Can you work these out from the model? Positions are in its coordinate system, mm. A direction names the side the tool comes from. Give positions to 0.01 mm unless a question says otherwise; leave off trailing zeros. Loops run counter-clockwise (first coordinate to the right, second up) from the corner with the lowest first, then second, coordinate; pieces in that order, holes last. Notation, with made-up numbers: (-24, 47.25) - (8, 47.25) arc R24 cw to (8, 76.25) - close; hole circle Ø10 at (-23, -33). An arc over 180 degrees is marked (long way). Write item = value, one per line.
from build123d import *

# Parameters (mm, degrees)
DELETE_START           = -13.5
DELETE_FACE_1_DEPTH    = 27
MOVE_FACE_1_BY         = 7
MOVE_FACE_2_BY         = 5.5
SKETCH_2_W             = 48.263019836
SKETCH_2_H             = 43.058184364
CUT_EXTRUDE_1_DEPTH    = 20
EXTRUDE_1_DEPTH        = 2
EXTRUDE_1_DEPTH_BACK   = 5
SKETCH_3_W             = 20
SKETCH_3_H             = 30
HOLE_WIZARD_M5_1_D     = 4.2
HOLE_WIZARD_M5_1_DEPTH = 20
HOLE_WIZARD_M5_1_TIP   = 1.2618073


with BuildPart() as part:
    # Delete Face 1: read off the stored shape, not the designer's step
    # Delete Face 1 outline → Delete Face 1 (new body)
    with BuildSketch(Plane.YZ.offset(DELETE_START)):
        with BuildLine():
            ThreePointArc((-8.364285714, 23.895568572), (-8.397831007, 23.931741933), (-8.41, 23.979551078))
            Line((-8.41, 23.979551078), (-8.41, 26.020448922))
            ThreePointArc((-8.41, 26.020448922), (-8.397831007, 26.068258067), (-8.364285714, 26.104431428))
            ThreePointArc((-8.364285714, 26.104431428), (-7.725958169, 26.423724028), (-7.033327746, 26.595982314))
            ThreePointArc((-7.033327746, 26.595982314), (-6.723611818, 26.762379014), (-6.6, 27.091517187))
            Line((-6.6, 27.091517187), (-6.6, 27.908482813))
            ThreePointArc((-6.6, 27.908482813), (-6.723615527, 28.237625227), (-7.033338915, 28.404019189))
            ThreePointArc((-7.033338915, 28.404019189), (-7.725963455, 28.576277924), (-8.364285714, 28.895568572))
            ThreePointArc((-8.364285714, 28.895568572), (-8.397831007, 28.931741933), (-8.41, 28.979551078))
            Line((-8.41, 28.979551078), (-8.41, 31.020448922))
            ThreePointArc((-8.41, 31.020448922), (-8.397831007, 31.068258067), (-8.364285714, 31.104431428))
            ThreePointArc((-8.364285714, 31.104431428), (-7.725958168, 31.423724029), (-7.033327744, 31.595982314))
            ThreePointArc((-7.033327744, 31.595982314), (-6.723611817, 31.762379015), (-6.6, 32.091517187))
            Line((-6.6, 32.091517187), (-6.6, 32.908482813))
            ThreePointArc((-6.6, 32.908482813), (-6.602116164, 32.954435895), (-6.608446743, 33))
            Line((-6.608446743, 33), (-12.6, 33))
            Line((-12.6, 33), (-12.6, -33))
            Line((-12.6, -33), (-6.608446743, -33))
            ThreePointArc((-6.608446743, -33), (-6.602116164, -32.954435895), (-6.6, -32.908482813))
            Line((-6.6, -32.908482813), (-6.6, -32.091517187))
            ThreePointArc((-6.6, -32.091517187), (-6.723615531, -31.762374768), (-7.033338927, -31.595980809))
            ThreePointArc((-7.033338927, -31.595980809), (-7.72596346, -31.423722074), (-8.364285714, -31.104431428))
            ThreePointArc((-8.364285714, -31.104431428), (-8.397831007, -31.068258067), (-8.41, -31.020448922))
            Line((-8.41, -31.020448922), (-8.41, -28.979551078))
            ThreePointArc((-8.41, -28.979551078), (-8.397831007, -28.931741933), (-8.364285714, -28.895568572))
            ThreePointArc((-8.364285714, -28.895568572), (-7.725958168, -28.576275971), (-7.033327744, -28.404017686))
            ThreePointArc((-7.033327744, -28.404017686), (-6.723611817, -28.237620985), (-6.6, -27.908482813))
            Line((-6.6, -27.908482813), (-6.6, -27.091517187))
            ThreePointArc((-6.6, -27.091517187), (-6.723615528, -26.762374772), (-7.033338917, -26.595980811))
            ThreePointArc((-7.033338917, -26.595980811), (-7.725963456, -26.423722076), (-8.364285714, -26.104431428))
            ThreePointArc((-8.364285714, -26.104431428), (-8.397831007, -26.068258067), (-8.41, -26.020448922))
            Line((-8.41, -26.020448922), (-8.41, -23.979551078))
            ThreePointArc((-8.41, -23.979551078), (-8.397831007, -23.931741933), (-8.364285714, -23.895568572))
            ThreePointArc((-8.364285714, -23.895568572), (-7.725958169, -23.576275972), (-7.033327746, -23.404017686))
            ThreePointArc((-7.033327746, -23.404017686), (-6.723611818, -23.237620986), (-6.6, -22.908482813))
            Line((-6.6, -22.908482813), (-6.6, -22.091517187))
            ThreePointArc((-6.6, -22.091517187), (-6.723615529, -21.76237477), (-7.033338921, -21.59598081))
            ThreePointArc((-7.033338921, -21.59598081), (-7.725963458, -21.423722075), (-8.364285714, -21.104431428))
            ThreePointArc((-8.364285714, -21.104431428), (-8.397831007, -21.068258067), (-8.41, -21.020448922))
            Line((-8.41, -21.020448922), (-8.41, -18.979551078))
            ThreePointArc((-8.41, -18.979551078), (-8.397831007, -18.931741933), (-8.364285714, -18.895568572))
            ThreePointArc((-8.364285714, -18.895568572), (-7.725958168, -18.576275971), (-7.033327744, -18.404017686))
            ThreePointArc((-7.033327744, -18.404017686), (-6.723611817, -18.237620985), (-6.6, -17.908482813))
            Line((-6.6, -17.908482813), (-6.6, -17.091517187))
            ThreePointArc((-6.6, -17.091517187), (-6.723615531, -16.762374768), (-7.033338926, -16.595980809))
            ThreePointArc((-7.033338926, -16.595980809), (-7.72596346, -16.423722074), (-8.364285714, -16.104431428))
            ThreePointArc((-8.364285714, -16.104431428), (-8.397831007, -16.068258067), (-8.41, -16.020448922))
            Line((-8.41, -16.020448922), (-8.41, -13.979551078))
            ThreePointArc((-8.41, -13.979551078), (-8.397831007, -13.931741933), (-8.364285714, -13.895568572))
            ThreePointArc((-8.364285714, -13.895568572), (-7.725958337, -13.576276034), (-7.033328102, -13.404017734))
            ThreePointArc((-7.033328102, -13.404017734), (-6.723611936, -13.237621121), (-6.6, -12.908482813))
            Line((-6.6, -12.908482813), (-6.6, -12.091517187))
            ThreePointArc((-6.6, -12.091517187), (-6.723615532, -11.762374767), (-7.033338929, -11.595980809))
            ThreePointArc((-7.033338929, -11.595980809), (-7.725963462, -11.423722074), (-8.364285714, -11.104431428))
            ThreePointArc((-8.364285714, -11.104431428), (-8.397831007, -11.068258067), (-8.41, -11.020448922))
            Line((-8.41, -11.020448922), (-8.41, -8.979551078))
            ThreePointArc((-8.41, -8.979551078), (-8.397831007, -8.931741933), (-8.364285714, -8.895568572))
            ThreePointArc((-8.364285714, -8.895568572), (-7.725958524, -8.576276103), (-7.033328496, -8.404017787))
            ThreePointArc((-7.033328496, -8.404017787), (-6.723612067, -8.23762127), (-6.6, -7.908482813))
            Line((-6.6, -7.908482813), (-6.6, -7.091517187))
            ThreePointArc((-6.6, -7.091517187), (-6.723615306, -6.762375026), (-7.033338249, -6.595980901))
            ThreePointArc((-7.033338249, -6.595980901), (-7.72596314, -6.423722193), (-8.364285714, -6.104431428))
            ThreePointArc((-8.364285714, -6.104431428), (-8.397831007, -6.068258067), (-8.41, -6.020448922))
            Line((-8.41, -6.020448922), (-8.41, -3.979551078))
            ThreePointArc((-8.41, -3.979551078), (-8.397831007, -3.931741933), (-8.364285714, -3.895568572))
            ThreePointArc((-8.364285714, -3.895568572), (-7.725958462, -3.57627608), (-7.033328366, -3.40401777))
            ThreePointArc((-7.033328366, -3.40401777), (-6.723612024, -3.237621221), (-6.6, -2.908482813))
            Line((-6.6, -2.908482813), (-6.6, -2.091517187))
            ThreePointArc((-6.6, -2.091517187), (-6.723615307, -1.762375024), (-7.033338252, -1.5959809))
            ThreePointArc((-7.033338252, -1.5959809), (-7.725963141, -1.423722192), (-8.364285714, -1.104431428))
            ThreePointArc((-8.364285714, -1.104431428), (-8.397831007, -1.068258067), (-8.41, -1.020448922))
            Line((-8.41, -1.020448922), (-8.41, 1.020448922))
            ThreePointArc((-8.41, 1.020448922), (-8.397831007, 1.068258067), (-8.364285714, 1.104431428))
            ThreePointArc((-8.364285714, 1.104431428), (-7.725958462, 1.42372392), (-7.033328366, 1.59598223))
            ThreePointArc((-7.033328366, 1.59598223), (-6.723612024, 1.762378779), (-6.6, 2.091517187))
            Line((-6.6, 2.091517187), (-6.6, 2.908482813))
            ThreePointArc((-6.6, 2.908482813), (-6.723615307, 3.237624975), (-7.033338252, 3.4040191))
            ThreePointArc((-7.033338252, 3.4040191), (-7.725963141, 3.576277808), (-8.364285714, 3.895568572))
            ThreePointArc((-8.364285714, 3.895568572), (-8.397831007, 3.931741933), (-8.41, 3.979551078))
            Line((-8.41, 3.979551078), (-8.41, 6.020448922))
            ThreePointArc((-8.41, 6.020448922), (-8.397831007, 6.068258067), (-8.364285714, 6.104431428))
            ThreePointArc((-8.364285714, 6.104431428), (-7.725958469, 6.423723918), (-7.03332838, 6.595982228))
            ThreePointArc((-7.03332838, 6.595982228), (-6.723612029, 6.762378774), (-6.6, 7.091517187))
            Line((-6.6, 7.091517187), (-6.6, 7.908482813))
            ThreePointArc((-6.6, 7.908482813), (-6.723615311, 8.23762498), (-7.033338263, 8.404019101))
            ThreePointArc((-7.033338263, 8.404019101), (-7.725963146, 8.57627781), (-8.364285714, 8.895568572))
            ThreePointArc((-8.364285714, 8.895568572), (-8.397831007, 8.931741933), (-8.41, 8.979551078))
            Line((-8.41, 8.979551078), (-8.41, 11.020448922))
            ThreePointArc((-8.41, 11.020448922), (-8.397831007, 11.068258067), (-8.364285714, 11.104431428))
            ThreePointArc((-8.364285714, 11.104431428), (-7.725958337, 11.423723966), (-7.033328101, 11.595982266))
            ThreePointArc((-7.033328101, 11.595982266), (-6.723611936, 11.76237888), (-6.6, 12.091517187))
            Line((-6.6, 12.091517187), (-6.6, 12.908482813))
            ThreePointArc((-6.6, 12.908482813), (-6.72361553, 13.237625231), (-7.033338924, 13.40401919))
            ThreePointArc((-7.033338924, 13.40401919), (-7.725963459, 13.576277925), (-8.364285714, 13.895568572))
            ThreePointArc((-8.364285714, 13.895568572), (-8.397831007, 13.931741933), (-8.41, 13.979551078))
            Line((-8.41, 13.979551078), (-8.41, 16.020448922))
            ThreePointArc((-8.41, 16.020448922), (-8.397831007, 16.068258067), (-8.364285714, 16.104431428))
            ThreePointArc((-8.364285714, 16.104431428), (-7.725958169, 16.423724029), (-7.033327745, 16.595982314))
            ThreePointArc((-7.033327745, 16.595982314), (-6.723611818, 16.762379015), (-6.6, 17.091517187))
            Line((-6.6, 17.091517187), (-6.6, 17.908482813))
            ThreePointArc((-6.6, 17.908482813), (-6.72361553, 18.23762523), (-7.033338923, 18.40401919))
            ThreePointArc((-7.033338923, 18.40401919), (-7.725963459, 18.576277925), (-8.364285714, 18.895568572))
            ThreePointArc((-8.364285714, 18.895568572), (-8.397831007, 18.931741933), (-8.41, 18.979551078))
            Line((-8.41, 18.979551078), (-8.41, 21.020448922))
            ThreePointArc((-8.41, 21.020448922), (-8.397831007, 21.068258067), (-8.364285714, 21.104431428))
            ThreePointArc((-8.364285714, 21.104431428), (-7.725958168, 21.423724029), (-7.033327744, 21.595982314))
            ThreePointArc((-7.033327744, 21.595982314), (-6.723611817, 21.762379015), (-6.6, 22.091517187))
            Line((-6.6, 22.091517187), (-6.6, 22.908482813))
            ThreePointArc((-6.6, 22.908482813), (-6.723615528, 23.237625227), (-7.033338915, 23.404019189))
            ThreePointArc((-7.033338915, 23.404019189), (-7.725963455, 23.576277924), (-8.364285714, 23.895568572))
        make_face()
    extrude(amount=DELETE_FACE_1_DEPTH)

    # Move Face 1: a face moved inward by 7.0
    extrude(part.faces().sort_by_distance((13.5, -10.05864991, 0))[0], amount=MOVE_FACE_1_BY, dir=(-1, 0, 0), mode=Mode.SUBTRACT)

    # Move Face 2: a face moved outward by 5.5
    extrude(part.faces().sort_by_distance((-3.5, -12.6, 0))[0], amount=MOVE_FACE_2_BY, dir=(0, -1, 0))

    # 草图2 → 切除-拉伸1 (cut)
    with BuildSketch(Plane.XZ.offset(18.1)):
        with Locations((-0.503276546, 38.529092182)):
            Rectangle(SKETCH_2_W, SKETCH_2_H)
    extrude(amount=-CUT_EXTRUDE_1_DEPTH, mode=Mode.SUBTRACT)

    # 草图3 → 凸台-拉伸1 (add, two sides: drawn at the far end of the back side and taken through both)
    with BuildSketch(Plane(origin=(0, -6.6, 0), x_dir=(1, 0, 0), z_dir=(0, 1, 0)).offset(-EXTRUDE_1_DEPTH_BACK)):
        with Locations((-3.5, -2)):
            Rectangle(SKETCH_3_W, SKETCH_3_H)
    extrude(amount=EXTRUDE_1_DEPTH + EXTRUDE_1_DEPTH_BACK)

    # M5 螺纹孔1
    with Locations(Plane(origin=(-4.186814404, -18.1, 12), x_dir=(0, 0, -1), z_dir=(0, -1, 0))):
        with Locations((0, 0), (18, 0)):
            Hole(HOLE_WIZARD_M5_1_D / 2, depth=HOLE_WIZARD_M5_1_DEPTH)
            with Locations((0, 0, -(HOLE_WIZARD_M5_1_DEPTH + HOLE_WIZARD_M5_1_TIP / 2))):  # 118° drill point
                Cone(0, HOLE_WIZARD_M5_1_D / 2, HOLE_WIZARD_M5_1_TIP, mode=Mode.SUBTRACT)


solid = part.part
Q1. For pin 1 (1 mm diameter, centred on x = 1.5, z = -19.5, fed in from +Y); pin 2 (1.6 mm diameter, centred on x = -8, z = -29.5, fed in from +Y); pin 3 (3.5 mm diameter, centred on x = -4.19, z = -6, fed in from -Y); pin 4 (0.9 mm diameter, centred on x = -7.5, z = -17.5, fed in from +Y), each with a flat end and sliding along its axis, tell me the tip position at first contact or that it passes through.
Output:
pin_1 = -8.41
pin_2 = -8.02
pin_3 = through
pin_4 = -6.6
Q2. I need wall thicknesses on L1, parallel to X at y = -9.5, z = -6; L2, parallel to Z at x = -4, y = -6.25; L3, parallel to Z at x = -10.5, y = -6.75. Which ranges of each line are inside material? Lowest first, please.
Output:
L1 = -13.5 to -6.29, -2.09 to 6.5
L2 = -13 to -8.09, -3.91 to 9.91, 14.09 to 17
L3 = -33 to -31.73, -28.27 to -26.73, -23.27 to -21.73, -18.27 to -16.73, -13.27 to 17
Q3. Imagine slicing it at D-D, the plane z = 10.5. Write out the boundary of the cut face in (x, y), then the cut area to 3 significant figures.
Output:
outline = (-13.5, -18.1) - (-5.66, -18.1) - (-5.66, -4.6) - (-13.5, -4.6) - close; (-2.72, -18.1) - (6.5, -18.1) - (6.5, -4.6) - (-2.72, -4.6) - close
area = 230 mm2
Q4. Imagine slicing it at B-B, the plane y = -5.5. Write out the boundary of the cut face in (x, z).
Output:
outline = (-13.5, -13) - (6.5, -13) - (6.5, 17) - (-13.5, 17) - close; hole circle Ø4.2 at (-4.19, -6); hole circle Ø4.2 at (-4.19, 12)
Q5. Which directions (+Z, -Z, +X, -X, +Y, -Y) give clear straight access to the entire face, cutting with the end or side of a thin tool? Please do faces 5 (the cylindrical face through (-3.64, -7.717, -31.427)), 6 (the flat face through (-4, -12, -33)).
Output:
face_5 = +X, -X, +Y
face_6 = -Z, +X, -X, +Y, -Y
Q6. Imagine slicing it at C-C, the plane x = -3.5. Give the number of separate pieces and of enclosed holes in the cut face, then the cut area to 3 significant figures.
Output:
separate_pieces = 3
enclosed_holes = 0
area = 507 mm2
Q7. Imagine slicing it at A-A, the plane z = -6. Write out the boundary of the cut face in (x, y).
Output:
outline = (-13.5, -18.1) - (-6.29, -18.1) - (-6.29, -4.6) - (-13.5, -4.6) - close; (-2.09, -18.1) - (6.5, -18.1) - (6.5, -4.6) - (-2.09, -4.6) - close
Q8. We'd pull the mould along Z, two halves only. Please class faces 1 (the flat face through (-13.5, -11, -8)), 2 (the flat face through (-4, -6, -13)), 3 (the flat face through (-4, -11, 17)), 4 (the flat face through (-4, -8.41, -15)): released by +Z, released by -Z, zero draft, split by the parting line, or undercut.
Output:
face_1 = zero draft
face_2 = released by -Z
face_3 = released by +Z
face_4 = undercut
